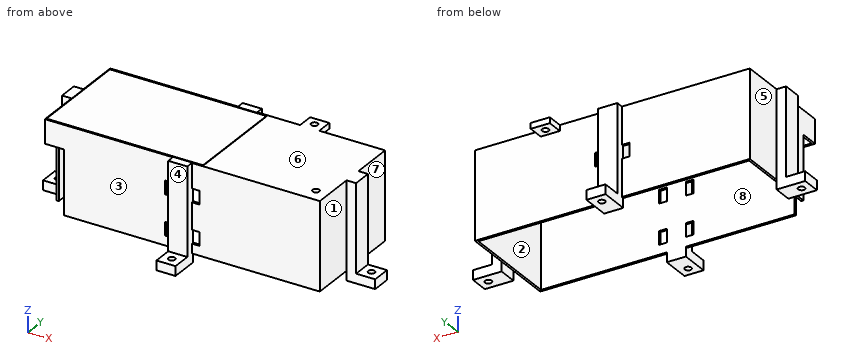
from build123d import *

# Parameters (mm, degrees)
SKETCH2_W             = 5
SKETCH2_H             = 10
BOSS_EXTRUDE1_DEPTH   = 48
SKETCH2_W_2           = 10
SKETCH2_H_2           = 5
BOSS_EXTRUDE1_2_DEPTH = 48
BOSS_EXTRUDE1_3_DEPTH = 48
BOSS_EXTRUDE1_4_DEPTH = 48
SKETCH3_W             = 165
SKETCH3_H             = 55.28
BOSS_EXTRUDE2_DEPTH   = 3
SKETCH4_W             = 10
SKETCH4_H             = 3.86
BOSS_EXTRUDE3_DEPTH   = 3
SKETCH5_W             = 10
SKETCH5_H             = 5
BOSS_EXTRUDE4_DEPTH   = 10
SKETCH7_W             = 5
SKETCH7_H             = 10
BOSS_EXTRUDE5_DEPTH   = 10
SKETCH8_R             = 1.73
CUT_EXTRUDE1_DEPTH    = 107.873978241
SKETCH10_W            = 10
SKETCH10_H            = 8.5
SKETCH10_W_2          = 1.85
SKETCH10_H_2          = 10
BOSS_EXTRUDE6_DEPTH   = 3
SKETCH11_R            = 1.75
CUT_EXTRUDE3_DEPTH    = 110.119417268
SKETCH12_W            = 82.72
SKETCH12_H            = 54.46
SKETCH12_W_2          = 81.92
SKETCH12_H_2          = 53.66
CUT_EXTRUDE4_DEPTH    = 0.28
CUT_EXTRUDE5_DEPTH    = 108.749929118
BOSS_EXTRUDE7_DEPTH   = 43
CUT_EXTRUDE6_DEPTH    = 33.5
SKETCH16_W            = 4
SKETCH16_H            = 7
CUT_EXTRUDE7_DEPTH    = 1.14
SKETCH17_W            = 4
SKETCH17_H            = 7
CUT_EXTRUDE8_DEPTH    = 1.14


with BuildPart() as part:
    # Sketch2 → Boss-Extrude1 (new body)
    with BuildSketch(Plane.XY):
        with Locations((-74.585, 0)):
            Rectangle(SKETCH2_W, SKETCH2_H)
    extrude(amount=BOSS_EXTRUDE1_DEPTH)



with BuildPart() as body_2:
    # Sketch2 → Boss-Extrude1 2 (new body)
    with BuildSketch(Plane.XY):
        with Locations((0, 29)):
            Rectangle(SKETCH2_W_2, SKETCH2_H_2)
    extrude(amount=BOSS_EXTRUDE1_2_DEPTH)


with BuildPart() as body_3:
    # Sketch2 → Boss-Extrude1 3 (new body)
    with BuildSketch(Plane.XY):
        with Locations((74.585, 0)):
            Rectangle(SKETCH2_W, SKETCH2_H)
    extrude(amount=BOSS_EXTRUDE1_3_DEPTH)


with BuildPart() as body_4:
    # Sketch2 → Boss-Extrude1 4 (new body)
    with BuildSketch(Plane.XY):
        with Locations((0, -29)):
            Rectangle(SKETCH2_W_2, SKETCH2_H_2)
    extrude(amount=BOSS_EXTRUDE1_4_DEPTH)


with BuildPart() as part_1:
    add(part.part)

    add(body_2.part)  # Boss-Extrude2 merges body 2

    add(body_3.part)  # Boss-Extrude2 merges body 3

    add(body_4.part)  # Boss-Extrude2 merges body 4
    # Sketch3 → Boss-Extrude2 (add)
    with BuildSketch(Plane.XY.offset(48)):
        Rectangle(SKETCH3_W, SKETCH3_H)
    extrude(amount=BOSS_EXTRUDE2_DEPTH)

    # Sketch4 → Boss-Extrude3 (add)
    with BuildSketch(Plane.XY.offset(48)):
        with Locations((0, 29.57)):
            Rectangle(SKETCH4_W, SKETCH4_H)
        with Locations((0, -29.57)):
            Rectangle(SKETCH4_W, SKETCH4_H)
    extrude(amount=BOSS_EXTRUDE3_DEPTH)

    # Sketch5 → Boss-Extrude4 (add)
    with BuildSketch(Plane(origin=(0, 5, 0), x_dir=(1, 0, 0), z_dir=(0, 1, 0))):
        with Locations((-82.085, -2.5)):
            Rectangle(SKETCH5_W, SKETCH5_H)
        with Locations((82.085, -2.5)):
            Rectangle(SKETCH5_W, SKETCH5_H)
    extrude(amount=-BOSS_EXTRUDE4_DEPTH)

    # Sketch7 → Boss-Extrude5 (add)
    with BuildSketch(Plane.ZY.offset(5)):
        with Locations((2.5, 36.5)):
            Rectangle(SKETCH7_W, SKETCH7_H)
        with Locations((2.5, -36.5)):
            Rectangle(SKETCH7_W, SKETCH7_H)
    extrude(amount=-BOSS_EXTRUDE5_DEPTH)

    # Sketch8 → Cut-Extrude1 (cut, through all)
    with BuildSketch(Plane.XY.offset(5)):
        with Locations((-82.085, 0)):
            Circle(SKETCH8_R)
        with Locations((0, -36.5)):
            Circle(SKETCH8_R)
        with Locations(Location((82.085, 0, 0), (0, 0, 180))):
            Circle(SKETCH8_R)
        with Locations(Location((0, 36.5, 0), (0, 0, 180))):
            Circle(SKETCH8_R)
    extrude(amount=-CUT_EXTRUDE1_DEPTH, mode=Mode.SUBTRACT)

    # Sketch10 → Boss-Extrude6 (add)
    with BuildSketch(Plane.XY.offset(51)):
        with Locations((32.52, 31.89)):
            Rectangle(SKETCH10_W, SKETCH10_H)
        with Locations((69.005, -20.32)):
            Rectangle(SKETCH10_W_2, SKETCH10_H_2)
    extrude(amount=-BOSS_EXTRUDE6_DEPTH)

    # Sketch11 → Cut-Extrude3 (cut, through all)
    with BuildSketch(Plane.XY.offset(51)):
        with Locations((32.52, 31.75)):
            Circle(SKETCH11_R)
        with Locations((65.54, -20.32)):
            Circle(SKETCH11_R)
    extrude(amount=-CUT_EXTRUDE3_DEPTH, mode=Mode.SUBTRACT)

    # Sketch12 → Cut-Extrude4 (cut)
    with BuildSketch(Plane.XY.offset(51)):
        with Locations((-30.625, 0)):
            Rectangle(SKETCH12_W, SKETCH12_H)
        with Locations((-30.625, 0)):
            Rectangle(SKETCH12_W_2, SKETCH12_H_2, mode=Mode.SUBTRACT)
    extrude(amount=-CUT_EXTRUDE4_DEPTH, mode=Mode.SUBTRACT)

    # Sketch13 → Cut-Extrude5 (cut, through all)
    with BuildSketch(Plane(origin=(0, 0, 48), x_dir=(-1, 0, 0), z_dir=(0, 0, -1))):
        Polygon((82.5, -27.64), (82.5, 27.64), (72.085, 27.64), (72.085, 5), (77.085, 5), (77.085, -5), (72.085, -5), (72.085, -27.64), align=None)
        Polygon((-82.5, 27.64), (-82.5, -27.64), (-72.085, -27.64), (-72.085, -5), (-77.085, -5), (-77.085, 5), (-72.085, 5), (-72.085, 27.64), align=None)
    extrude(amount=-CUT_EXTRUDE5_DEPTH, mode=Mode.SUBTRACT)

    # Sketch14 → Boss-Extrude7 (add)
    with BuildSketch(Plane(origin=(0, 0, 48), x_dir=(-1, 0, 0), z_dir=(0, 0, -1))):
        Polygon((72.085, -27.64), (5, -27.64), (5, -26.5), (70.945, -26.5), (70.945, -5), (70.945, 5), (70.945, 26.5), (5, 26.5), (5, 27.64), (72.085, 27.64), (72.085, 5), (72.085, -5), align=None)
        Polygon((-72.085, 5), (-72.085, -5), (-72.085, -27.64), (-5, -27.64), (-5, -26.5), (-70.945, -26.5), (-70.945, -5), (-70.945, 5), (-70.945, 26.5), (-37.52, 26.5), (-27.52, 26.5), (-5, 26.5), (-5, 27.64), (-27.52, 27.64), (-37.52, 27.64), (-72.085, 27.64), align=None)
    extrude(amount=BOSS_EXTRUDE7_DEPTH)

    # Sketch15 → Cut-Extrude6 (cut)
    with BuildSketch(Plane(origin=(0, 0, 5), x_dir=(-1, 0, 0), z_dir=(0, 0, -1))):
        Polygon((72.085, -17.64), (70.945, -17.64), (70.945, -26.5), (62.085, -26.5), (62.085, -27.64), (72.085, -27.64), align=None)
    extrude(amount=-CUT_EXTRUDE6_DEPTH, mode=Mode.SUBTRACT)

    # Sketch16 → Cut-Extrude7 (cut)
    with BuildSketch(Plane.XZ.offset(27.64)):
        with Locations((7, 34.5)):
            Rectangle(SKETCH16_W, SKETCH16_H)
        with Locations((7, 13.5)):
            Rectangle(SKETCH16_W, SKETCH16_H)
        with Locations((-7, 13.5)):
            Rectangle(SKETCH16_W, SKETCH16_H)
        with Locations((-7, 34.5)):
            Rectangle(SKETCH16_W, SKETCH16_H)
    extrude(amount=-CUT_EXTRUDE7_DEPTH, mode=Mode.SUBTRACT)

    # Sketch17 → Cut-Extrude8 (cut)
    with BuildSketch(Plane(origin=(0, 27.64, 0), x_dir=(1, 0, 0), z_dir=(0, 1, 0))):
        with Locations((7, -28)):
            Rectangle(SKETCH17_W, SKETCH17_H)
        with Locations((-7, -28)):
            Rectangle(SKETCH17_W, SKETCH17_H)
    extrude(amount=-CUT_EXTRUDE8_DEPTH, mode=Mode.SUBTRACT)


solid = part_1.part
Source: CAD feature listing. Evaluate the final solid. Frame: model axes, mm. Face numbers are marked on the shaded views. A direction names the side the tool comes from. Give positions to 0.01 mm unless a question says otherwise; leave off trailing zeros. Write each loop counter-clockwise with the first axis right and the second up, starting at its lowest first coordinate (ties: lowest second). Pieces come first, ordered by that corner, then holes. Notation, with made-up numbers: M -40,56 L 16,56 A17 ccw 16,61 Z; hole C 37.5,-13.5 d7. An arc over 180 degrees is marked long. Answer as a JSON object with one key per item and string values.
Q1. Cut plane B-B, the plane y = -20.32. Return the cut outline in (x, z) (3 decimals), then the cut area to 3 significant figures.
Geometry check:
{"outline": "M -72.085,38.5 L -70.945,38.5 L -70.945,48 L 63.79,48 L 63.79,51 L 10.735,51 L 10.735,50.72 L 10.335,50.72 L 10.335,51 L -71.585,51 L -71.585,50.72 L -71.985,50.72 L -71.985,51 L -72.085,51 Z; M 67.29,48 L 70.945,48 L 70.945,5 L 72.085,5 L 72.085,51 L 67.29,51 Z", "area": "482 mm^2"}
Q2. Cut plane C-C, the plane x = 32.52. Return the cut outline in (y, z).
Geometry check:
{"outline": "M -27.64,5 L -26.5,5 L -26.5,48 L 26.5,48 L 26.5,5 L 27.64,5 L 27.64,48 L 30,48 L 30,51 L -27.64,51 Z; M 33.5,48 L 36.14,48 L 36.14,51 L 33.5,51 Z"}
Q3. Cut plane A-A, the plane z = 29. Count the separate pieces of the cut face and the enclosed holes in it, then the cut area to 3 significant figures.
Geometry check:
{"separate pieces": "3", "enclosed holes": "0", "area": "596 mm^2"}
Q4. Mould query, pull axis X, two halves, no side actions, for the marked faces 6, 7 and 8. Classes: +X half, -X half, draft (parallel to the pull), parting line (faces both ways), or undercut.
Geometry check:
{"face 6": "draft", "face 7": "+X half", "face 8": "undercut"}
Q5. Ray query, line 1 along Y through (x, z) = (33, 17.5); line 2 along X through (y, z) = (36.5, 2.15); line 3 along X through (y, z) = (23, 11.5) (3 decimals). Return the intervals inside material, ascending.
Geometry check:
{"line 1": "y = -27.64 to -26.5, 26.5 to 27.64", "line 2": "x = -5 to -1.73, 1.73 to 5", "line 3": "x = -72.085 to -70.945, 70.945 to 72.085"}
Q6. Access query for the marked faces 1, 2, 3, 4 and 5. Directions: +Z, -Z, +X, -X, +Y, -Y. A direction counts if a zero-diameter tool reaches every point of the face in a straight line with its end or side. Return the directions, or none.
Geometry check:
{"face 1": "+Z, -Z, +X, -Y", "face 2": "-Z", "face 3": "+Z, -Z, -X, -Y", "face 4": "+Z, +X, -X, -Y", "face 5": "+Z, -Z, -X, +Y"}
Q7. Cut plane D-D, the plane x = 0. Return the cut outline in (y, z), then the cut area to 3 significant figures.
Geometry check:
{"outline": "M -41.5,0 L -38.23,0 L -38.23,5 L -41.5,5 Z; M -34.77,0 L -26.5,0 L -26.5,48 L 26.5,48 L 26.5,0 L 34.77,0 L 34.77,5 L 31.5,5 L 31.5,51 L 27.23,51 L 27.23,50.72 L 26.83,50.72 L 26.83,51 L -26.83,51 L -26.83,50.72 L -27.23,50.72 L -27.23,51 L -31.5,51 L -31.5,5 L -34.77,5 Z; M 38.23,0 L 41.5,0 L 41.5,5 L 38.23,5 Z", "area": "734 mm^2"}
Q8. Contact query for flat-ended pins moving along their axis: P1, Ø3, axis at x = -66, y = 15, coming from the -Z side; P2, Ø4, axis at y = 23.5, z = 29.5, coming from the -X side (3 decimals); P3, Ø11, axis at x = 0, y = 34.5, coming from the +Z side; P4, Ø1, axis at x = 42.5, z = 28.5, coming from the -Y side. Output: stop coordinate, or through.
Geometry check:
{"P1": "stops at z = 48", "P2": "stops at x = -72.085", "P3": "stops at z = 51", "P4": "stops at y = -27.64"}
